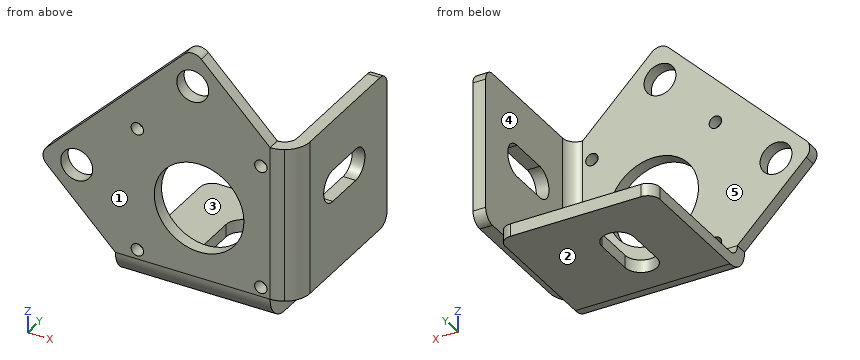
from build123d import *

# Parameters (mm, degrees)
SKETCH2_W                    = 42
SKETCH2_H                    = 42
BOSS_EXTRUDE1_DEPTH          = 3.175
SKETCH3_R                    = 11.25
SKETCH3_R_2                  = 1.554126588
CUT_EXTRUDE1_DEPTH           = 3.175
EDGE_FLANGE3_STRIP_W         = 19.05
EDGE_FLANGE3_STRIP_H         = 3.175
EDGE_FLANGE3_STRIP_CUT_DEPTH = 42
EDGE_FLANGE3_DEPTH           = 42
EDGE_FLANGE4_START           = -24.175
EDGE_FLANGE4_OUTLINE_W       = 3.175
EDGE_FLANGE4_OUTLINE_H       = 6.35
EDGE_FLANGE4_DEPTH           = 6.35
EDGE_FLANGE4_START_2         = -17.825
EDGE_FLANGE4_2_DEPTH         = 38.825
EDGE_FLANGE4_3_DEPTH         = 38.825
SKETCH22_W                   = 3.175
SKETCH22_H                   = 33.65
CUT_EXTRUDE2_DEPTH           = 3.175
SKETCH23_R                   = 4
BOSS_EXTRUDE2_DEPTH          = 3.175
CUT_EXTRUDE3_REACH           = 88.051
FILLET1_R                    = 3


# Read off the part's stored shape, not the designer's step: Edge-Flange4
# Sheet-metal steps are written as plain solids
with BuildPart() as part:
    # Sketch2 → Boss-Extrude1 (new body)
    with BuildSketch(Plane(origin=(0, 0, 0), x_dir=(1, 0, 0), z_dir=(0, 1, 0))):
        Rectangle(SKETCH2_W, SKETCH2_H)
    extrude(amount=BOSS_EXTRUDE1_DEPTH)

    # Sketch3 → Cut-Extrude1 (cut)
    with BuildSketch(Plane(origin=(0, 3.175, 0), x_dir=(1, 0, 0), z_dir=(0, 1, 0))):
        with Locations(Location((0, 0, 0), (0, 0, 270))):
            Circle(SKETCH3_R)
        with Locations(Location((-15.494, 15.494, 0), (0, 0, 270))):
            Circle(SKETCH3_R_2)
        with Locations(Location((15.494, 15.494, 0), (0, 0, 270))):
            Circle(SKETCH3_R_2)
        with Locations(Location((15.494, -15.494, 0), (0, 0, 270))):
            Circle(SKETCH3_R_2)
        with Locations(Location((-15.494, -15.494, 0), (0, 0, 270))):
            Circle(SKETCH3_R_2)
    extrude(amount=-CUT_EXTRUDE1_DEPTH, mode=Mode.SUBTRACT)

    # Edge-Flange3 strip (across the edge) → Edge-Flange3 strip cut (cut)
    with BuildSketch(Plane(origin=(21, 3.175, -21), x_dir=(0, 0, 1), z_dir=(-1, 0, 0))):
        with Locations((-6.35, -1.5875)):
            Rectangle(EDGE_FLANGE3_STRIP_W, EDGE_FLANGE3_STRIP_H)
    extrude(amount=EDGE_FLANGE3_STRIP_CUT_DEPTH, mode=Mode.SUBTRACT)

    # Edge-Flange3 section (across the edge) → Edge-Flange3 (add)
    with BuildSketch(Plane(origin=(21, 3.175, -21), x_dir=(0, 0, 1), z_dir=(-1, 0, 0))):
        with BuildLine():
            Line((-3.175, 3.175), (-3.175, 36.825))
            Line((-3.175, 36.825), (0, 36.825))
            Line((0, 36.825), (0, 3.175))
            ThreePointArc((0, 3.175), (0.92993597, 0.92993597), (3.175, 0))
            Line((3.175, 0), (3.175, -3.175))
            ThreePointArc((3.175, -3.175), (-1.315128061, -1.315128061), (-3.175, 3.175))
        make_face()
    extrude(amount=EDGE_FLANGE3_DEPTH)

    # Edge-Flange4 outline → Edge-Flange4 (cut)
    with BuildSketch(Plane.XY.offset(EDGE_FLANGE4_START)):
        with Locations((19.4125, 3.175)):
            Rectangle(EDGE_FLANGE4_OUTLINE_W, EDGE_FLANGE4_OUTLINE_H)
    extrude(amount=EDGE_FLANGE4_DEPTH, mode=Mode.SUBTRACT)

    # Edge-Flange4 2 outline → Edge-Flange4 2 (cut)
    with BuildSketch(Plane.XY.offset(EDGE_FLANGE4_START_2)):
        with BuildLine():
            ThreePointArc((21, 0.850738685), (19.468500936, 0.216371003), (17.825, 0))
            Line((17.825, 0), (21, 0))
            Line((21, 0), (21, 0.850738685))
        make_face()
    extrude(amount=EDGE_FLANGE4_2_DEPTH, mode=Mode.SUBTRACT)

    # Edge-Flange4 3 outline → Edge-Flange4 3 (add)
    with BuildSketch(Plane.XY.offset(EDGE_FLANGE4_START_2)):
        with BuildLine():
            Line((17.825, 3.175), (21, 3.175))
            Line((21, 3.175), (21, 0.850738685))
            ThreePointArc((21, 0.850738685), (23.324261314, 3.174999999), (24.175, 6.35))
            Line((24.175, 6.35), (24.175, 40))
            Line((24.175, 40), (21, 40))
            Line((21, 40), (21, 6.35))
            ThreePointArc((21, 6.35), (20.07006403, 4.10493597), (17.825, 3.175))
        make_face()
    extrude(amount=EDGE_FLANGE4_3_DEPTH)

    # Sketch22 → Cut-Extrude2 (cut)
    with BuildSketch(Plane(origin=(0, 0, -24.175), x_dir=(-1, 0, 0), z_dir=(0, 0, -1))):
        with Locations((-19.4125, 23.175)):
            Rectangle(SKETCH22_W, SKETCH22_H)
    extrude(amount=-CUT_EXTRUDE2_DEPTH, mode=Mode.SUBTRACT)

    # Sketch23 → Boss-Extrude2 (add)
    # profile 1 of 2: a face of its own
    with BuildSketch(Plane(origin=(0, 3.175, 0), x_dir=(1, 0, 0), z_dir=(0, 1, 0))):
        Polygon((-21, -21), (-21, 17.825), (-40.4125, -1.5875), align=None)
        with Locations(Location((-30.70625, -1.5875, 0), (0, 0, 270))):
            Circle(SKETCH23_R, mode=Mode.SUBTRACT)
    # profile 2 of 2: a face of its own
    with BuildSketch(Plane(origin=(0, 3.175, 0), x_dir=(1, 0, 0), z_dir=(0, 1, 0))):
        Polygon((17.825, -21), (-21, -21), (-1.5875, -40.4125), align=None)
        with Locations(Location((-1.5875, -30.70625, 0), (0, 0, 270))):
            Circle(SKETCH23_R, mode=Mode.SUBTRACT)
    extrude(amount=-BOSS_EXTRUDE2_DEPTH)

    # Sketch24 → Cut-Extrude3 (cut, up to next)
    with BuildSketch(Plane(origin=(0, 0, -24.175), x_dir=(-1, 0, 0), z_dir=(0, 0, -1)), mode=Mode.PRIVATE) as cut_extrude3_sk1:
        with BuildLine():
            Line((0.4, 16.35), (0.4, 26.35))
            ThreePointArc((0.4, 26.35), (4.4, 30.35), (8.4, 26.35))
            Line((8.4, 26.35), (8.4, 16.35))
            ThreePointArc((8.4, 16.35), (4.4, 12.35), (0.4, 16.35))
        make_face()
    cut_extrude3_tool1 = extrude(cut_extrude3_sk1.sketch, amount=-CUT_EXTRUDE3_REACH, mode=Mode.PRIVATE) & part.part
    cut_extrude3 = cut_extrude3_tool1.solids().sort_by_distance((-4.4, 21.35, -24.175))[0]
    add(cut_extrude3, mode=Mode.SUBTRACT)

    # Mirror1: Cut-Extrude3 across plane
    add(cut_extrude3.mirror(Plane(origin=(0, 0, 0), x_dir=(-0.7071067811865478, 2.4649279095086426e-15, 0.7071067811865472), z_dir=(-0.7071067811865475, 2.4649279095086418e-15, -0.7071067811865477))), mode=Mode.SUBTRACT)

    # Fillet1
    fillet1_edges = [part.edges().sort_by_distance(p)[0] for p in [
        (-40.4125, 1.5875, 1.5875),
        (-1.5875, 1.5875, 40.4125),
        (-21, 40, -22.5875),
        (22.5875, 40, 21),
        (22.5875, 40, -17.825),
        (17.825, 40, -22.5875),
    ]]
    fillet(fillet1_edges, radius=FILLET1_R)


solid = part.part
Geometry: final body of the model. Coordinates: model frame, mm. Face numbers are marked on the shaded views. A direction names the side the tool comes from. Give positions to 0.01 mm unless a question says otherwise; leave off trailing zeros. Write each loop counter-clockwise with the first axis right and the second up, starting at its lowest first coordinate (ties: lowest second). Pieces come first, ordered by that corner, then holes. Notation, with made-up numbers: (81, 71) -> (134, 71) arc R32 cw to (134, 103) -> close; hole circle Ø8 at (-26, 46.5). An arc over 180 degrees is marked (long way). Answer as a JSON object with one key per item and string values.
1. Cut plane C-C on x = 8.5. Output: boundary loops of the cut face in (y, z) (3 decimals).
Ans:
{"outline": "(0, -17.825) arc R6.35 ccw to (6.35, -24.175) -> (40, -24.175) -> (40, -21) -> (6.35, -21) arc R3.175 cw to (3.175, -17.825) -> (3.175, -7.37) -> (0, -7.37) -> close; (0, 7.37) -> (3.175, 7.37) -> (3.175, 30.325) -> (0, 30.325) -> close"}
2. Cut plane A-A on y = 19. Output: boundary loops of the cut face in (x, z) (3 decimals).
Ans:
{"outline": "(-21, -24.175) -> (-8.4, -24.175) -> (-8.4, -21) -> (-21, -21) -> close; (-0.4, -24.175) -> (17.825, -24.175) -> (17.825, -21) -> (-0.4, -21) -> close; (21, -17.825) -> (24.175, -17.825) -> (24.175, 0.4) -> (21, 0.4) -> close; (21, 8.4) -> (24.175, 8.4) -> (24.175, 21) -> (21, 21) -> close"}
3. Ray query, probe 1 along X at (y, z) = (11.5, -10.5) (3 decimals); probe 2 along Y at (x, z) = (-7, 14.5) (3 decimals); probe 3 along Z at (x, y) = (8, 34.5) (3 decimals). Return the intervals inside material, ascending. Write a range as from..to.
Ans:
{"probe 1": "x = 21..24.175", "probe 2": "y = 0..3.175", "probe 3": "z = -24.175..-21"}
4. Cut plane D-D on z = 12.5. Output: boundary loops of the cut face in (x, y) (3 decimals), and give its area (3 significant figures).
Ans:
{"outline": "(-29.5, 0) -> (17.825, 0) arc R6.35 ccw to (24.175, 6.35) -> (24.175, 40) -> (21, 40) -> (21, 6.35) arc R3.175 cw to (17.825, 3.175) -> (-29.5, 3.175) -> close", "area": "281 mm^2"}
5. Contact query for flat-ended pins moving along their axis: pin 1 (5 mm diameter, centred on x = -28.5, z = -14, fed in from +Y); pin 2 (6 mm diameter, centred on x = -11.5, z = 31, fed in from +Y) (3 decimals); pin 3 (1 mm diameter, centred on x = 22, y = 22, fed in from -Z) (3 decimals); pin 4 (6 mm diameter, centred on y = 5, z = -6, fed in from -X). Output: stop coordinate, or through.
Ans:
{"pin 1": "passes through", "pin 2": "stops at y = 3.175", "pin 3": "stops at z = -17.825", "pin 4": "stops at x = -35.21"}
6. Access query for the marked faces 1, 2, 3, 4 and 5. Directions: +Z, -Z, +X, -X, +Y, -Y. A direction counts if a zero-diameter tool reaches every point of the face in a straight line with its end or side. Return the directions, or none.
Ans:
{"face 1": "+Z, -Z, +X, -X, -Y", "face 2": "-Z, +X, -X, +Y, -Y", "face 3": "+Z, +X, -X, +Y", "face 4": "+Z, -Z, -X, +Y", "face 5": "+Z, -X, +Y"}
7. Cut plane B-B on y = 11. Output: boundary loops of the cut face in (x, z) (3 decimals), and give its area (3 significant figures).
Ans:
{"outline": "(-21, -24.175) -> (17.825, -24.175) -> (17.825, -21) -> (-21, -21) -> close; (21, -17.825) -> (24.175, -17.825) -> (24.175, 21) -> (21, 21) -> close", "area": "247 mm^2"}
